from build123d import *

# Parameters (mm, degrees)
SKETCH_1_W      = 230
SKETCH_1_H      = 230
SKETCH_1_R      = 1.5
SKETCH_1_R_2    = 2
EXTRUDE_1_DEPTH = 12
CHAMFER_1_SIZE  = 2
CHAMFER_2_SIZE  = 2.2


with BuildPart() as part:
    # Эскиз1 → Бобышка-Вытянуть1 (new body)
    with BuildSketch(Plane.XY):
        with Locations((115, 115)):
            Rectangle(SKETCH_1_W, SKETCH_1_H)
        with Locations((219.5, 10.5)):
            Circle(SKETCH_1_R, mode=Mode.SUBTRACT)
        with Locations((219.5, 219.5)):
            Circle(SKETCH_1_R, mode=Mode.SUBTRACT)
        with Locations((10.5, 219.5)):
            Circle(SKETCH_1_R, mode=Mode.SUBTRACT)
        with Locations((10.5, 10.5)):
            Circle(SKETCH_1_R, mode=Mode.SUBTRACT)
        with Locations((115, 219.5)):
            Circle(SKETCH_1_R, mode=Mode.SUBTRACT)
        with Locations((225, 150)):
            Circle(SKETCH_1_R_2, mode=Mode.SUBTRACT)
        with Locations((225, 210)):
            Circle(SKETCH_1_R_2, mode=Mode.SUBTRACT)
    extrude(amount=EXTRUDE_1_DEPTH)

    # Фаска1
    chamfer_1_edges = [part.edges().sort_by_distance(p)[0] for p in [
        (218, 10.5, 12),
        (218, 219.5, 12),
        (9, 219.5, 12),
        (9, 10.5, 12),
        (113.5, 219.5, 12),
    ]]
    chamfer(chamfer_1_edges, length=CHAMFER_1_SIZE)

    # Фаска2
    chamfer_2_edges = [part.edges().sort_by_distance(p)[0] for p in [
        (223, 150, 12),
        (223, 210, 12),
    ]]
    chamfer(chamfer_2_edges, length=CHAMFER_2_SIZE)


solid = part.part
Could you check a few things on this model? Use its own coordinates, in mm. Round coordinates to 2 decimals unless told otherwise and drop trailing zeros.
Q1. Thinking about a two-plate mould opening in X: for faces 1 (the face through (230, 113, 6)), 2 (the face through (113, 230, 6)), 3 (the face through (114.65, 217.91, 10.13)), which applies, released by +X, released by -X, zero draft, split by the parting line, or undercut?
Geometry says:
face 1: released by +X
face 2: zero draft
face 3: undercut
Q2. Please list where these lines run through material, in increasing order: probe 1 along X at (y, z) = (219.5, 5.25); probe 2 along Y at (x, z) = (219.5, 7); probe 3 along X at (y, z) = (210, 3).
Geometry says:
probe 1: x = 0 to 9, 12 to 113.5, 116.5 to 218, 221 to 230
probe 2: y = 0 to 9, 12 to 218, 221 to 230
probe 3: x = 0 to 223, 227 to 230
Q3. I'm going to push flat-ended pins straight in: P1, Ø1.8, axis at x = 10.5, y = 219.5, coming from the +Z side; P2, Ø5, axis at x = 170.5, y = 88, coming from the -Z side. Where does each tip first touch, or does it pass through?
Geometry says:
P1: passes through
P2: stops at z = 0
